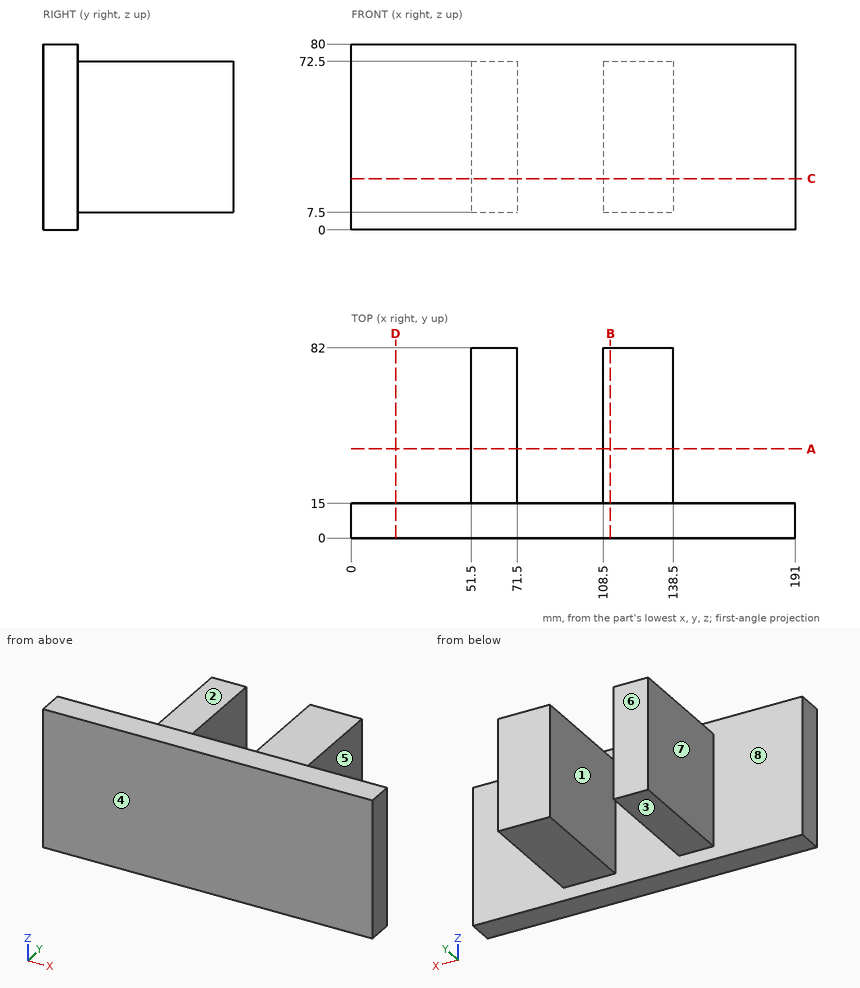
Could you check a few things on this drawing? It's one solid part, dimensions in mm from its lowest x, y, z. A direction names the side the tool comes from. Round coordinates to 2 decimals unless told otherwise and drop trailing zeros. Loops run counter-clockwise (first coordinate to the right, second up) from the corner with the lowest first, then second, coordinate; pieces in that order, holes last.
Q1. Thinking about a two-plate mould opening in X: for the marked faces 5, 6, 7 and 8, which applies, pulls with the +X half, pulls with the -X half, needs draft (parallel to the pull), parting line crosses it, or undercut?
Q2. I want a section at B-B (x = 111.5). Write out the boundary of the cut face in (y, z).
Q3. I want a section at A-A (y = 38.5). Write out the boundary of the cut face in (x, z).
Q4. I want a section at D-D (x = 19). Write out the boundary of the cut face in (y, z), and give its area (3 significant figures).
Q5. Please list where these lines run through material, in increasing order: L1, parallel to X at y = 43, z = 53; L2, parallel to Y at x = 80.5, z = 66.
Q6. I want a section at C-C (z = 22). Write out the boundary of the cut face in (x, y).
Q7. For P1, Ø24, axis at x = 95.5, z = 59.5, coming from the +Y side; P2, Ø2, axis at y = 23, z = 29.5, coming from the +X side; P3, Ø22, axis at x = 62, y = 40, coming from the -Z side, each with a flat end and sliding along its axis, tell me the tip position at first contact or that it passes through.
Q8. On a 3-axis mill with a long thin cutter (end or side, diameter ignored), from which of +Z, -Z, +X, -X, +Y, -Y can I reach the whole of each face in a straight line? I mean the marked faces 1, 2, 3 and 4. Say none if no direction works.
Answer below:
1. face 5: pulls with the +X half
1. face 6: needs draft
1. face 7: pulls with the -X half
1. face 8: undercut
2. outline: (0, 0) - (15, 0) - (15, 7.5) - (82, 7.5) - (82, 72.5) - (15, 72.5) - (15, 80) - (0, 80) - close
3. outline: (51.5, 7.5) - (71.5, 7.5) - (71.5, 72.5) - (51.5, 72.5) - close; (108.5, 7.5) - (138.5, 7.5) - (138.5, 72.5) - (108.5, 72.5) - close
4. outline: (0, 0) - (15, 0) - (15, 80) - (0, 80) - close
4. area: 1,200 mm2
5. L1: x = 51.5 to 71.5, 108.5 to 138.5
5. L2: y = 0 to 15
6. outline: (0, 0) - (191, 0) - (191, 15) - (138.5, 15) - (138.5, 82) - (108.5, 82) - (108.5, 15) - (71.5, 15) - (71.5, 82) - (51.5, 82) - (51.5, 15) - (0, 15) - close
7. P1: stops at y = 15
7. P2: stops at x = 138.5
7. P3: stops at z = 7.5
8. face 1: +Z, -Z, +Y
8. face 2: +Z, +X, -X, +Y
8. face 3: -Z, +X, -X, +Y
8. face 4: +Z, -Z, +X, -X, -Y
